Check sheet for the modelled part. Datum: model origin and axes. Units: mm. A direction names the side the tool comes from. Coordinates: 2 decimals unless noted, no trailing zeros. Loops run counter-clockwise (first coordinate to the right, second up) from the corner with the lowest first, then second, coordinate; pieces in that order, holes last. Notation, with made-up numbers: M -2.5,40.5 L 18.5,40.5 A6 cw 18.5,49.5 Z; hole C -1,-31 d7. An arc over 180 degrees is marked long. Return JSON: item names as keys, results as strings.
from build123d import *

# Parameters (mm, degrees)
BOSS_EXTRUDE1_START     = 33.3375
SKETCH1_R               = 12.7
BOSS_EXTRUDE1_DEPTH     = 4.7625
BOSS_EXTRUDE2_START     = -38.1
SKETCH1_6_R             = 12.7
BOSS_EXTRUDE2_DEPTH     = 4.7625
BOSS_EXTRUDE3_DEPTH     = 33.3375
BOSS_EXTRUDE4_START     = -38.1
BOSS_EXTRUDE4_DEPTH     = 38.1
SKETCH2_W               = 66.675
SKETCH2_H               = 67.807583187
CUT_EXTRUDE1_DEPTH      = 4.7625
SKETCH3_R               = 2.603499999
CUT_EXTRUDE2_DEPTH      = 4.7625
SKETCH4_R               = 2.6035
SKETCH4_R_2             = 2.603499999
CUT_EXTRUDE3_DEPTH      = 4.7625
SKETCH5_R               = 2.6035
SKETCH5_R_2             = 3.2639
CUT_EXTRUDE4_DEPTH      = 688.71544222
CUT_EXTRUDE5_DEPTH      = 685.541963263
CUT_EXTRUDE5_DEPTH_BACK = 685.541963263
SKETCH6_R               = 2.6035
SKETCH7_R               = 9.525
CUT_EXTRUDE6_DEPTH      = 688.71544222
FILLET1_R               = 4.7625
SKETCH8_W               = 9.525
SKETCH8_H               = 6.35
CUT_EXTRUDE7_DEPTH      = 9.525


with BuildPart() as part:
    # Sketch1 → Boss-Extrude1 (new body)
    with BuildSketch(Plane(origin=(0, 0, 0), x_dir=(0, 0, -1), z_dir=(1, 0, 0)).offset(BOSS_EXTRUDE1_START)):
        with BuildLine():
            Line((41.306573009, 186.931527045), (41.306573009, 644.131527045))
            ThreePointArc((41.306573009, 644.131527045), (3.206573009, 682.231527045), (-34.893426991, 644.131527045))
            Line((-34.893426991, 644.131527045), (-34.893426991, 186.931527045))
            ThreePointArc((-34.893426991, 186.931527045), (3.206573009, 148.831527045), (41.306573009, 186.931527045))
        make_face()
        with Locations((3.206573009, 186.931527045)):
            Circle(SKETCH1_R, mode=Mode.SUBTRACT)
        with Locations((3.206573009, 644.131527045)):
            Circle(SKETCH1_R, mode=Mode.SUBTRACT)
    extrude(amount=BOSS_EXTRUDE1_DEPTH)

    # Sketch1<7> → Boss-Extrude3 (add)
    with BuildSketch(Plane(origin=(0, 0, 0), x_dir=(0, 0, -1), z_dir=(1, 0, 0))):
        with BuildLine():
            ThreePointArc((-34.893426991, 186.931527045), (-33.683593364, 177.406527045), (-30.130926991, 168.486443859))
            Line((-30.130926991, 168.486443859), (-30.130926991, 662.576610232))
            ThreePointArc((-30.130926991, 662.576610232), (-33.683593364, 653.656527045), (-34.893426991, 644.131527045))
            Line((-34.893426991, 644.131527045), (-34.893426991, 186.931527045))
        make_face()
        with BuildLine():
            ThreePointArc((36.544073009, 168.486443859), (40.096739381, 177.406527045), (41.306573009, 186.931527045))
            Line((41.306573009, 186.931527045), (41.306573009, 644.131527045))
            ThreePointArc((41.306573009, 644.131527045), (40.096739381, 653.656527045), (36.544073009, 662.576610232))
            Line((36.544073009, 662.576610232), (36.544073009, 168.486443859))
        make_face()
    extrude(amount=BOSS_EXTRUDE3_DEPTH)



with BuildPart() as body_2:
    # Sketch1<6> → Boss-Extrude2 (new body)
    with BuildSketch(Plane(origin=(0, 0, 0), x_dir=(0, 0, -1), z_dir=(1, 0, 0)).offset(BOSS_EXTRUDE2_START)):
        with BuildLine():
            Line((41.306573009, 186.931527045), (41.306573009, 644.131527045))
            ThreePointArc((41.306573009, 644.131527045), (3.206573009, 682.231527045), (-34.893426991, 644.131527045))
            Line((-34.893426991, 644.131527045), (-34.893426991, 186.931527045))
            ThreePointArc((-34.893426991, 186.931527045), (3.206573009, 148.831527045), (41.306573009, 186.931527045))
        make_face()
        with Locations(Location((3.206573009, 186.931527045, 0), (0, 0, 180))):
            Circle(SKETCH1_6_R, mode=Mode.SUBTRACT)
        with Locations(Location((3.206573009, 644.131527045, 0), (0, 0, 180))):
            Circle(SKETCH1_6_R, mode=Mode.SUBTRACT)
    extrude(amount=BOSS_EXTRUDE2_DEPTH)


with BuildPart() as part_1:
    add(part.part)

    add(body_2.part)  # Boss-Extrude4 merges body 2
    # Sketch1<8> → Boss-Extrude4 (add)
    with BuildSketch(Plane(origin=(0, 0, 0), x_dir=(0, 0, -1), z_dir=(1, 0, 0)).offset(BOSS_EXTRUDE4_START)):
        with BuildLine():
            ThreePointArc((-34.893426991, 186.931527045), (-33.683593364, 177.406527045), (-30.130926991, 168.486443859))
            Line((-30.130926991, 168.486443859), (-30.130926991, 662.576610232))
            ThreePointArc((-30.130926991, 662.576610232), (-33.683593364, 653.656527045), (-34.893426991, 644.131527045))
            Line((-34.893426991, 644.131527045), (-34.893426991, 186.931527045))
        make_face()
        with BuildLine():
            ThreePointArc((36.544073009, 168.486443859), (40.096739381, 177.406527045), (41.306573009, 186.931527045))
            Line((41.306573009, 186.931527045), (41.306573009, 644.131527045))
            ThreePointArc((41.306573009, 644.131527045), (40.096739381, 653.656527045), (36.544073009, 662.576610232))
            Line((36.544073009, 662.576610232), (36.544073009, 168.486443859))
        make_face()
    extrude(amount=BOSS_EXTRUDE4_DEPTH)

    # Sketch2 → Cut-Extrude1 (cut)
    with BuildSketch(Plane.XY.offset(34.893426991)):
        with Locations((0, 628.672818639)):
            Rectangle(SKETCH2_W, SKETCH2_H)
    extrude(amount=-CUT_EXTRUDE1_DEPTH, mode=Mode.SUBTRACT)

    # Sketch3 → Cut-Extrude2 (cut)
    with BuildSketch(Plane.XY.offset(34.893426991)):
        with Locations((23, 575.769027045)):
            Circle(SKETCH3_R)
        with Locations((23, 588.769027045)):
            Circle(SKETCH3_R)
        with Locations((-23, 575.769027045)):
            Circle(SKETCH3_R)
        with Locations((-23, 588.769027045)):
            Circle(SKETCH3_R)
        with Locations((-23, 230.269027045)):
            Circle(SKETCH3_R)
        with Locations((23, 230.269027045)):
            Circle(SKETCH3_R)
    extrude(amount=-CUT_EXTRUDE2_DEPTH, mode=Mode.SUBTRACT)

    # Sketch4 → Cut-Extrude3 (cut)
    with BuildSketch(Plane(origin=(0, 0, -41.306573009), x_dir=(-1, 0, 0), z_dir=(0, 0, -1))):
        with Locations(Location((-23, 205.631527043, 0), (0, 0, 90))):
            Circle(SKETCH4_R)
        with Locations(Location((-23, 218.631527043, 0), (0, 0, 90))):
            Circle(SKETCH4_R)
        with Locations(Location((23, 218.631527043, 0), (0, 0, 90))):
            Circle(SKETCH4_R)
        with Locations(Location((23, 205.631527043, 0), (0, 0, 90))):
            Circle(SKETCH4_R)
        with Locations(Location((23, 614.131527045, 0), (0, 0, 90))):
            Circle(SKETCH4_R_2)
        with Locations(Location((-23, 614.131527045, 0), (0, 0, 90))):
            Circle(SKETCH4_R_2)
    extrude(amount=-CUT_EXTRUDE3_DEPTH, mode=Mode.SUBTRACT)

    # Sketch5 → Cut-Extrude4 (cut, through all)
    with BuildSketch(Plane.ZY.offset(38.1)):
        with Locations(Location((-3.206573009, 352.031527045, 0), (0, 0, 270))):
            Circle(SKETCH5_R)
        with Locations(Location((-3.206573009, 402.831527045, 0), (0, 0, 270))):
            Circle(SKETCH5_R)
        with Locations(Location((-3.206573009, 377.431527045, 0), (0, 0, 270))):
            Circle(SKETCH5_R_2)
    extrude(amount=-CUT_EXTRUDE4_DEPTH, mode=Mode.SUBTRACT)

    # Sketch6 → Cut-Extrude5 (cut, two sides: drawn at the far end of the back side and taken through both)
    with BuildSketch(Plane(origin=(0, 0, 0), x_dir=(0, 0, -1), z_dir=(1, 0, 0)).offset(-CUT_EXTRUDE5_DEPTH_BACK)):
        with Locations((25.431573009, 186.931527045)):
            Circle(SKETCH6_R)
        with Locations((3.206573009, 209.156527045)):
            Circle(SKETCH6_R)
        with Locations((-19.018426991, 186.931527045)):
            Circle(SKETCH6_R)
        with Locations((3.206573009, 164.706527045)):
            Circle(SKETCH6_R)
        with Locations((-19.018426991, 644.131527045)):
            Circle(SKETCH6_R)
        with Locations((3.206573009, 666.356527045)):
            Circle(SKETCH6_R)
        with Locations((25.431573009, 644.131527045)):
            Circle(SKETCH6_R)
        with Locations((3.206573009, 621.906527045)):
            Circle(SKETCH6_R)
    extrude(amount=CUT_EXTRUDE5_DEPTH + CUT_EXTRUDE5_DEPTH_BACK, mode=Mode.SUBTRACT)

    # Sketch7 → Cut-Extrude6 (cut, through all)
    with BuildSketch(Plane(origin=(38.1, 0, 0), x_dir=(0, 0, -1), z_dir=(1, 0, 0))):
        with Locations((25.431573009, 209.156527045)):
            Circle(SKETCH7_R)
        with Locations(Location((25.431573009, 621.906527045, 0), (0, 0, 270))):
            Circle(SKETCH7_R)
        with Locations(Location((-19.018426991, 209.156527045, 0), (0, 0, 270))):
            Circle(SKETCH7_R)
        with Locations((-19.018426991, 621.906527045)):
            Circle(SKETCH7_R)
    extrude(amount=-CUT_EXTRUDE6_DEPTH, mode=Mode.SUBTRACT)

    # Fillet1
    fillet1_edges = [part_1.edges().sort_by_distance(p)[0] for p in [
        (-33.3375, 594.769027045, 32.512176991),
        (33.3375, 594.769027045, 32.512176991),
    ]]
    fillet(fillet1_edges, radius=FILLET1_R)

    # Sketch8 → Cut-Extrude7 (cut)
    with BuildSketch(Plane.ZY.offset(38.1)):
        with Locations((-36.544073009, 606.031527045)):
            Rectangle(SKETCH8_W, SKETCH8_H)
        with Locations((-36.544073009, 593.331527045)):
            Rectangle(SKETCH8_W, SKETCH8_H)
        with Locations((-36.544073009, 529.831527045)):
            Rectangle(SKETCH8_W, SKETCH8_H)
        with Locations((-36.544073009, 517.131527045)):
            Rectangle(SKETCH8_W, SKETCH8_H)
    cut_extrude7 = extrude(amount=-CUT_EXTRUDE7_DEPTH, mode=Mode.SUBTRACT)

    # Mirror1: Cut-Extrude7 across plane
    add(cut_extrude7.mirror(Plane(origin=(0, 0, 0), x_dir=(0, 0, 1), z_dir=(1, 0, 0))), mode=Mode.SUBTRACT)


solid = part_1.part
1) Set-up check for faces 4 (the face through (38.1, 419, -3)), 5 (the face through (-35.685, 631.422, -25.85)), 6 (the face through (0, 381, 30.131)), 7 (the face through (-34, 596.507, -38)), 8 (the face through (34, 609.207, -38)): record each of +Z, -Z, +X, -X, +Y, -Y from which the full face is reachable in a straight line by a thin tool's end or side.
Answers:
{"face 4": "+Z, -Z, +X, +Y, -Y", "face 5": "+X, -X", "face 6": "+Y, -Y", "face 7": "-Z, -X", "face 8": "-Z, +X"}
2) Section check B-B on y = 559. Record the cut outline in (x, z).
Answers:
{"outline": "M -38.1,-41.31 L 38.1,-41.31 L 38.1,34.89 L -38.1,34.89 Z; hole M -33.34,-36.54 L 33.34,-36.54 L 33.34,30.13 L -33.34,30.13 Z"}
3) Section check A-A on x = -14. Record the cut outline in (y, z).
Answers:
{"outline": "M 168.49,-36.54 A38.1 ccw 186.93,-41.31 L 644.13,-41.31 A38.1 ccw 662.58,-36.54 Z; M 168.49,30.13 L 594.77,30.13 L 594.77,34.89 L 186.93,34.89 A38.1 ccw Z"}
4) Scan lines: line 1 along X through (y, z) = (301, 20.5); line 2 along Z through (x, y) = (-10, 436); line 3 along Y through (x, z) = (-33.5, -30). Record each from-to range of solid material in increasing order. Write a range as [from, to].
Answers:
{"line 1": "[-38.1, -33.34], [33.34, 38.1]", "line 2": "[-41.31, -36.54], [30.13, 34.89]", "line 3": "[159.84, 200.8], [217.51, 613.55], [630.26, 671.22]"}
5) Go/stop test with flat-tipped pins: pin 1 Ø4.5 at (y, z) = (209.16, -3.21) entering from +X; pin 2 Ø10.5 at (y, z) = (377.43, -3.21) entering from -X; pin 3 Ø10 at (x, z) = (28.5, -15) entering from -Y; pin 4 Ø7.5 at (x, z) = (-35.5, -34.5) entering from +Y. Record where each tip stops, or that it passes through.
Answers:
{"pin 1": "through", "pin 2": "x = -38.1", "pin 3": "y = 150.32", "pin 4": "y = 670.46"}
6) Draft check along Z on faces 1 (the face through (-9, 181.14, 34.45)), 2 (the face through (34, 602.857, -38)), 3 (the face through (-35.69, 200.71, -29.83)). Enter one of: +Z half, -Z half, draft (parallel to the pull), parting line (faces both ways), or undercut.
Answers:
{"face 1": "parting line", "face 2": "draft", "face 3": "undercut"}
